Solid Edge part; units mm, degrees
sketch "Sketch1" plane through (0, 0, 0) normal (0, 0, 1) x (1, 0, 0)
  line L0 (19.4702, 0) -> (45, 0)
  line L1 (45, 1) -> (45, 0)
  line L2 (19.4702, 1) -> (45, 1)
  arc A0 (17.4936, 2.6954) -> (19.4702, 1) centre (19.4702, 3) ccw
  arc A1 (-17.4936, 2.6954) -> (17.4936, 2.6954) centre (0, 0) cw
  arc A2 (-19.4702, 1) -> (-17.4936, 2.6954) centre (-19.4702, 3) ccw
  line L3 (-45, 1) -> (-19.4702, 1)
  line L4 (-45, 1) -> (-45, 0)
  line L5 (-45, 0) -> (-19.4702, 0)
  arc A3 (-19.4702, 0) -> (-16.5052, 2.5431) centre (-19.4702, 3) ccw
  arc A4 (16.5052, 2.5431) -> (19.4702, 0) centre (19.4702, 3) ccw
  arc A5 (-16.5052, 2.5431) -> (16.5052, 2.5431) centre (0, 0) cw
extrude "Protrusion1" add sketch "Sketch1" along normal blind 20
sketch "Sketch2" plane through (-32.2351, 1, 10) normal (0, 1, 0) x (-1, 0, 0)
  circle A0 centre (2.7649, 0) radius 5
  circle A1 centre (-67.2351, 0) radius 5
extrude "Cutout1" cut sketch "Sketch2" against normal up to next
fillet "Round_1" radius 5 4 edges at (-45, 0.5, 20) (-45, 0.5, 0) (45, 0.5, 20) (45, 0.5, 0)
properties material "Steel, structural"
The model under review builds one solid part; all positions refer to its coordinate system, in mm. A direction names the side the tool comes from. Round coordinates to 2 decimals unless told otherwise and drop trailing zeros. Write each loop counter-clockwise with the first axis right and the second up, starting at its lowest first coordinate (ties: lowest second). Pieces come first, ordered by that corner, then holes. Notation, with made-up numbers: M 62.25,0 L 112.25,0 A13 ccw 112.25,18 Z; hole C 43.5,64 d4. An arc over 180 degrees is marked long. Use a Markdown table: item, result. Add a question column.
Q1. We need section B-B, the plane z = 10. State the section outline as (x, y) points, plus the area to 3 significant figures.
Q2. We need section D-D, the plane z = 13.75. State the section outline as (x, y) points.
Q3. We need section A-A, the plane x = 35. State the section outline as (y, z) points.
Q4. To check wall thickness, follow line 1 (Z direction, x = -35, y = 0.55); line 2 (Y direction, x = -30, z = 5.5); line 3 (X direction, y = 3, z = 11.5). State the ranges of each line that lie inside material, in increasing order.
Q5. The part is to be moulded in two halves that separate along Z. For faces 1 (the face through (39.995, 0.507, 10.22)), 2 (the face through (-43.57, 0.49, 1.5)), 3 (the face through (-0.351, 17.697, 9.86)), say which applies: pulls with the +Z half, pulls with the -Z half, needs draft (parallel to the pull), parting line crosses it, or undercut.
Q6. Machinability: for faces 4 (the face through (29, 1, 10)), 5 (the face through (-29.6, 1, 9.9)), 6 (the face through (17.54, 0.704, 9.86)), which of the approach directions +Z, -Z, +X, -X, +Y, -Y give a long, thin tool a straight path to every point of the face, cutting with its end or side? Answer none if there is none.
Q7. We need section C-C, the plane y = 13.5. State the section outline as (x, z) points.
Q8. Insertion check: pin 1 (10 mm diameter, centred on x = 18, y = 15, fed in from -Z); pin 2 (6 mm diameter, centred on x = 35, z = 13.5, fed in from +Y); pin 3 (2 mm diameter, centred on y = 2.5, z = 6, fed in from -X). Each pin has a flat end and moves straight along its axis. Give the tip position at first contact, or say it passes through.
Findings below:
| question | item | result |
|---|---|---|
| 1 | outline | M -45,0 L -40,0 L -40,1 L -45,1 Z; M -30,0 L -19.47,0 A3 ccw -16.51,2.54 A16.7 cw 16.51,2.54 A3 ccw 19.47,0 L 30,0 L 30,1 L 19.47,1 A2 cw 17.49,2.7 A17.7 ccw -17.49,2.7 A2 cw -19.47,1 L -30,1 Z; M 40,0 L 45,0 L 45,1 L 40,1 Z |
| 1 | area | 86.9 mm² |
| 2 | outline | M -45,0 L -38.31,0 L -38.31,1 L -45,1 Z; M -31.69,0 L -19.47,0 A3 ccw -16.51,2.54 A16.7 cw 16.51,2.54 A3 ccw 19.47,0 L 31.69,0 L 31.69,1 L 19.47,1 A2 cw 17.49,2.7 A17.7 ccw -17.49,2.7 A2 cw -19.47,1 L -31.69,1 Z; M 38.31,0 L 45,0 L 45,1 L 38.31,1 Z |
| 3 | outline | M 0,0 L 1,0 L 1,5 L 0,5 Z; M 0,15 L 1,15 L 1,20 L 0,20 Z |
| 4 | line 1 | z = 0 to 5, 15 to 20 |
| 4 | line 2 | y = 0 to 1 |
| 4 | line 3 | x = -17.44 to -16.43, 16.43 to 17.44 |
| 5 | face 1 | undercut |
| 5 | face 2 | pulls with the -Z half |
| 5 | face 3 | needs draft |
| 6 | face 4 | +Z, -Z, +X, +Y |
| 6 | face 5 | +Z, -Z, -X, +Y |
| 6 | face 6 | +Z, -Z, -Y |
| 7 | outline | M -11.45,0 L -9.83,0 L -9.83,20 L -11.45,20 Z; M 9.83,0 L 11.45,0 L 11.45,20 L 9.83,20 Z |
| 8 | pin 1 | passes through |
| 8 | pin 2 | stops at y = 1 |
| 8 | pin 3 | stops at x = -18.15 |
